```python
from build123d import *

# Parameters (mm, degrees)
F0_W     = 52.226100117
F0_H     = 51.8441870809
F1_DEPTH = 50.8
F2_R     = 9.1837080102
F3_DEPTH = 58.674
F4_W     = 25.969831273
F4_H     = 25.969831273
F5_DEPTH = 12.7
F6_R     = 11.765038499
F7_DEPTH = 12.7


with BuildPart() as f1:
    # F0 (on Top) → F1 (new body)
    with BuildSketch(Plane.XY):
        with Locations((26.1130500585, 25.9220935404)):
            Rectangle(F0_W, F0_H)
    extrude(amount=F1_DEPTH)

    # F2 (on face) → F3 (cut)
    with BuildSketch(Plane.XY.offset(50.8)):
        with Locations((22.0552645624, 26.8291290849)):
            Circle(F2_R)
    extrude(amount=-F3_DEPTH, mode=Mode.SUBTRACT)

    # F4 (on face) → F5 (join)
    with BuildSketch(Plane(origin=(0, 51.8441870809, 0), x_dir=(-1, 0, 0), z_dir=(0, 1, 0))):
        with Locations((-27.7839014307, 31.9849038497)):
            Rectangle(F4_W, F4_H)
    extrude(amount=F5_DEPTH)

    # F6 (on face) → F7 (join)
    with BuildSketch(Plane(origin=(0, 0, 0), x_dir=(0, -1, 0), z_dir=(-1, 0, 0))):
        with Locations((-31.2210861593, 25.1105371863)):
            Circle(F6_R)
    extrude(amount=F7_DEPTH)


solid = f1.part
```
Geometry: final body of the model. Coordinates: model frame, mm. A direction names the side the tool comes from. Coordinates: 2 decimals unless noted, no trailing zeros. Loops run counter-clockwise (first coordinate to the right, second up) from the corner with the lowest first, then second, coordinate; pieces in that order, holes last. Notation, with made-up numbers: (51, 39.25) -> (67, 39.25) arc R23 ccw to (67, 53.25) -> close; hole circle Ø3 at (72, 70). An arc over 180 degrees is marked (long way). Use a Markdown table: item, result. Add a question column.
(1) Mould query, pull axis X, two halves, no side actions, for faces 1 (the cylindrical face through (14.8, 21.2, 25.8)), 2 (the flat face through (26, 51.844, 14)), 3 (the flat face through (14.799, 58, 32)). Classes: pulls with the +X half, pulls with the -X half, needs draft (parallel to the pull), parting line crosses it, or undercut.
(2) Section query B-B, the plane y = 31.5. Return loops of the section in (x, z), plus the area to 3 significant figures.
(3) Pin query (flat end, axial travel): pin 1 Ø10 at (y, z) = (60.5, 34.5) entering from +X; pin 2 Ø10 at (y, z) = (60.5, 36.5) entering from -X; pin 3 Ø1 at (y, z) = (20, 12) entering from -X. Return the tip coordinate at first contact, or that it passes through.
(4) Section query A-A, the plane x = 26.5. Return loops of the section in (y, z), plus the area to 3 significant figures.
(5) Access query for faces 4 (the flat face through (28, 58, 19)), 5 (the flat face through (0, 20, 31)), 6 (the flat face through (40.769, 58, 32)), 7 (the flat face through (28, 58, 44.97)). Directions: +Z, -Z, +X, -X, +Y, -Y. A direction counts if a zero-diameter tool reaches every point of the face in a straight line with its end or side. Return the directions, or none.
(6) Section query D-D, the plane y = 38. Return loops of the section in (x, z).
(7) Section query C-C, the plane z = 23. Return loops of the section in (x, y), plus the area to 3 significant figures.
(8) Line query: line 1 along X through (y, z) = (37.5, 8.5); line 2 along X through (y, z) = (28, 22.5); line 3 along Y through (x, z) = (49, 30). Output: solid intervals per line, ascending.
Answer:
| question | item | result |
|---|---|---|
| 1 | face 1 | undercut |
| 1 | face 2 | needs draft |
| 1 | face 3 | pulls with the -X half |
| 2 | outline | (-12.7, 13.35) -> (0, 13.35) -> (0, 0) -> (14.15, 0) -> (14.15, 50.8) -> (0, 50.8) -> (0, 36.87) -> (-12.7, 36.87) -> close; (29.96, 0) -> (52.23, 0) -> (52.23, 50.8) -> (29.96, 50.8) -> close |
| 2 | area | 2,150 mm^2 |
| 3 | pin 1 | stops at x = 40.77 |
| 3 | pin 2 | stops at x = 14.8 |
| 3 | pin 3 | stops at x = 0 |
| 4 | outline | (0, 0) -> (18.79, 0) -> (18.79, 50.8) -> (0, 50.8) -> close; (34.87, 0) -> (51.84, 0) -> (51.84, 19) -> (64.54, 19) -> (64.54, 44.97) -> (51.84, 44.97) -> (51.84, 50.8) -> (34.87, 50.8) -> close |
| 4 | area | 2,150 mm^2 |
| 5 | face 4 | -Z, +X, -X, +Y |
| 5 | face 5 | -X |
| 5 | face 6 | +Z, -Z, +X, +Y |
| 5 | face 7 | +Z, +X, -X, +Y |
| 6 | outline | (-12.7, 15.49) -> (0, 15.49) -> (0, 0) -> (52.23, 0) -> (52.23, 50.8) -> (0, 50.8) -> (0, 34.73) -> (-12.7, 34.73) -> close |
| 7 | outline | (-12.7, 19.65) -> (0, 19.65) -> (0, 0) -> (52.23, 0) -> (52.23, 51.84) -> (40.77, 51.84) -> (40.77, 64.54) -> (14.8, 64.54) -> (14.8, 51.84) -> (0, 51.84) -> (0, 42.8) -> (-12.7, 42.8) -> close; hole circle Ø18.37 at (22.06, 26.83) |
| 7 | area | 3,070 mm^2 |
| 8 | line 1 | x = 0 to 52.23 |
| 8 | line 2 | x = -12.7 to 12.95, 31.16 to 52.23 |
| 8 | line 3 | y = 0 to 51.84 |
